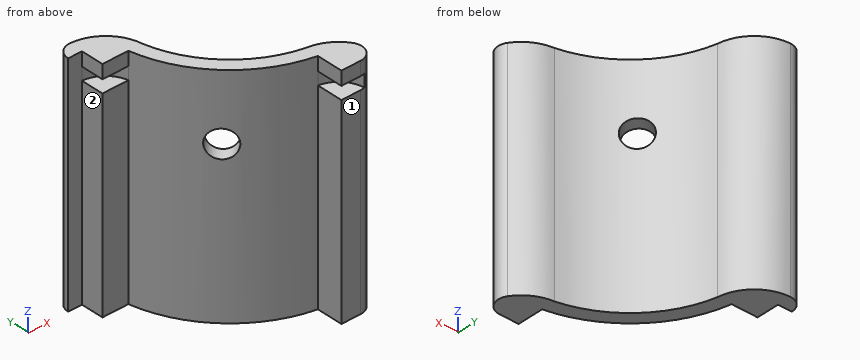
from build123d import *

# Parameters (mm, degrees)
BOSS_EXTRUDE1_DEPTH = 104.775
BOSS_EXTRUDE2_DEPTH = 92.5957
BOSS_EXTRUDE3_START = -5.8293
BOSS_EXTRUDE3_DEPTH = 5.8293
BOSS_EXTRUDE4_DEPTH = 6.35
SKETCH5_W           = 7.787485422
SKETCH5_H           = 19.833751934
SKETCH5_W_2         = 22.754058967
SKETCH5_H_2         = 3.407024872
CUT_EXTRUDE1_DEPTH  = 227.312030137
SKETCH6_R           = 6.35
CUT_EXTRUDE2_DEPTH  = 6.35
SKETCH7_W           = 111.054240747
SKETCH7_H           = 89.646194338
CUT_EXTRUDE3_DEPTH  = 104.775
SKETCH8_W           = 104.775
SKETCH8_H           = 6.354337814
BOSS_EXTRUDE5_DEPTH = 6.35
FILLET1_R           = 6.35


with BuildPart() as part:
    # Sketch1 → Boss-Extrude1 (new, symmetric)
    with BuildSketch(Plane.XY):
        with BuildLine():
            Line((-58.2422, 56.2102), (-58.2422, 62.5602))
            ThreePointArc((-58.2422, 62.5602), (-45.640852469, 57.743322347), (-39.3748699, 45.7962))
            ThreePointArc((-39.3748699, 45.7962), (-25.556268964, 20.239931036), (0, 6.4213301))
            ThreePointArc((0, 6.4213301), (12.247457496, 0.293755183), (17.272, -12.446))
            Line((17.272, -12.446), (10.922, -12.446))
            ThreePointArc((10.922, -12.446), (7.760938146, -4.204686933), (0, 0))
            ThreePointArc((0, 0), (-30.011530905, 15.784669095), (-45.7962, 45.7962))
            ThreePointArc((-45.7962, 45.7962), (-50.144819563, 53.243313205), (-58.2422, 56.2102))
        make_face()
    extrude(amount=BOSS_EXTRUDE1_DEPTH, both=True)


with BuildPart() as boss_extrude2_tool:
    # Sketch2 → Boss-Extrude2 (new, symmetric)
    with BuildSketch(Plane.XY):
        with BuildLine():
            Line((-58.2422, 56.2102), (-58.2422, 45.796198296))
            Line((-58.2422, 45.796198296), (-45.796199685, 45.796198296))
            ThreePointArc((-45.796199685, 45.796198296), (-50.144818899, 53.243312648), (-58.2422, 56.2102))
        make_face()
        with BuildLine():
            Line((0, 0), (0, -12.446))
            Line((0, -12.446), (10.922, -12.446))
            ThreePointArc((10.922, -12.446), (7.760938146, -4.204686933), (0, 0))
        make_face()
    extrude(amount=BOSS_EXTRUDE2_DEPTH, both=True)


with BuildPart() as part_1:
    add(part.part)


with BuildPart() as part_2:
    # Boss-Extrude2: joined with boss_extrude2_tool
    add(part_1.part.fuse(boss_extrude2_tool.part, tol=0.00001))

    # Sketch3 → Boss-Extrude3 (add)
    with BuildSketch(Plane(origin=(0, 0, -104.775), x_dir=(-1, 0, 0), z_dir=(0, 0, -1)).offset(BOSS_EXTRUDE3_START)):
        with BuildLine():
            Line((58.2422, 56.2102), (58.2422, 45.796198296))
            Line((58.2422, 45.796198296), (45.7962, 45.7962))
            ThreePointArc((45.7962, 45.7962), (50.144819563, 53.243313205), (58.2422, 56.2102))
        make_face()
        with BuildLine():
            Line((0, 0), (0, -12.446))
            Line((0, -12.446), (-10.922, -12.446))
            ThreePointArc((-10.922, -12.446), (-7.760938146, -4.204686933), (0, 0))
        make_face()
    extrude(amount=BOSS_EXTRUDE3_DEPTH)

    # Sketch4 → Boss-Extrude4 (add)
    with BuildSketch(Plane.XY.offset(104.775)):
        with BuildLine():
            Line((-58.2422, 56.2102), (-58.2422, 45.796198296))
            Line((-58.2422, 45.796198296), (-45.7962, 45.7962))
            ThreePointArc((-45.7962, 45.7962), (-50.144819563, 53.243313205), (-58.2422, 56.2102))
        make_face()
        with BuildLine():
            Line((0, 0), (0, -12.446))
            Line((0, -12.446), (10.922, -12.446))
            ThreePointArc((10.922, -12.446), (7.760938146, -4.204686933), (0, 0))
        make_face()
    extrude(amount=-BOSS_EXTRUDE4_DEPTH)

    # Sketch5 → Cut-Extrude1 (cut, through all)
    with BuildSketch(Plane.XY.offset(104.775)):
        with Locations((-61.627942711, 54.680509116)):
            Rectangle(SKETCH5_W, SKETCH5_H)
        with Locations((8.225058429, -13.641512436)):
            Rectangle(SKETCH5_W_2, SKETCH5_H_2)
    extrude(amount=-CUT_EXTRUDE1_DEPTH, mode=Mode.SUBTRACT)

    # Sketch6 → Cut-Extrude2 (cut, symmetric)
    with BuildSketch(Plane(origin=(-5.969, -5.969000176, 0), x_dir=(-0.7071067916239179, 0.7071067707491772, 0), z_dir=(-0.7071067707491772, -0.7071067916239179, 0))):
        with Locations(Location((32.382802858, -74.165398348, 0), (0, 0, 180))):
            Circle(SKETCH6_R)
    extrude(amount=CUT_EXTRUDE2_DEPTH, both=True, mode=Mode.SUBTRACT)

    # Sketch7 → Cut-Extrude3 (cut)
    with BuildSketch(Plane(origin=(0, 0, -104.775), x_dir=(-1, 0, 0), z_dir=(0, 0, -1))):
        with Locations((26.053941981, 26.416451063)):
            Rectangle(SKETCH7_W, SKETCH7_H)
    extrude(amount=-CUT_EXTRUDE3_DEPTH, mode=Mode.SUBTRACT)

    # Sketch8 → Boss-Extrude5 (add)
    with BuildSketch(Plane.ZY.offset(57.7342)):
        with Locations((52.3875, 59.374341949)):
            Rectangle(SKETCH8_W, SKETCH8_H)
    extrude(amount=BOSS_EXTRUDE5_DEPTH)

    # Fillet1
    # the kernel refuses this fillet: 6.35 mm, written as the material it takes off along each edge
    with BuildSketch(Plane(origin=(-64.0842, 62.551510856, -15.875), x_dir=(1, 0, 0), z_dir=(0, 0, 1))) as fillet1_piece_1:
        with BuildLine():
            CenterArc((FILLET1_R, -FILLET1_R), FILLET1_R, 90, 90)
            Line((0, -FILLET1_R), (0, 0))
            Line((0, 0), (FILLET1_R, 0))
        make_face()
    extrude(amount=136.525, mode=Mode.SUBTRACT)
    with BuildSketch(Plane(origin=(17.260151367, -11.938, -25.849178653), x_dir=(-0.30497213299383213, 0.9523612749882223, 0), z_dir=(0, 0, 1))) as fillet1_piece_2:
        with BuildLine():
            CenterArc((8.625598356, 6.114282737), FILLET1_R, 162.243512631, 123.416753829)
            Line((2.57810426, 8.050855782), (0, 0))
            ThreePointArc((0, 0), (5.169835731, -0.710949564), (10.339671461, 0))
        make_face()
    extrude(amount=156.473357306, mode=Mode.SUBTRACT)


solid = part_2.part
Work out the finished part from the listing and answer in its coordinate system (mm). Face numbers are marked on the shaded views. A direction names the side the tool comes from. Round coordinates to 2 decimals unless told otherwise and drop trailing zeros. Loops run counter-clockwise (first coordinate to the right, second up) from the corner with the lowest first, then second, coordinate; pieces in that order, holes last. Notation, with made-up numbers: (-16.75, 70.5) - (16.25, 70.5) arc R8 cw to (16.25, 83.5) - close; hole circle Ø9 at (53.5, 63). An arc over 180 degrees is marked (long way). One line per item, written item: value.
Q1. For the marked faces 1 and 2, determine the directions among +Z, -Z, +X, -X, +Y, -Y from which every point of the face is accessible in a straight line to the end or side of a thin tool.
Check values:
face 1: +Z, -Z, +X, -X, -Y
face 2: +Z, -Z, -X, -Y
Q2. Straight lines are drawn through the part: probe 1 along Y at (x, z) = (-23.5, 54); probe 2 along Y at (x, z) = (-35, 32.5); probe 3 along X at (y, z) = (37.5, 88). For each, find the intervals that lie inside material, in ascending order.
Check values:
probe 1: 10.19 to 18.3
probe 2: 21.48 to 33.29
probe 3: -43.61 to -36.89
Q3. Find section B-B on x = -48. Give the vertices of the cut face in (y, z) (3 decimals).
Check values:
outline: (45.796, 0) - (59.532, 0) - (59.532, 104.775) - (45.796, 104.775) - (45.796, 98.425) - (50.942, 98.425) - (50.942, 92.596) - (45.796, 92.596) - close
Q4. Find section C-C on y = 52.5. Give the vertices of the cut face in (x, z) (3 decimals), and give its area (3 significant figures).
Check values:
outline: (-57.734, 0) - (-41.501, 0) - (-41.501, 104.775) - (-57.734, 104.775) - (-57.734, 98.425) - (-49.331, 98.425) - (-49.331, 92.596) - (-57.734, 92.596) - close
area: 1,650 mm2
Q5. Each of these flat-tipped pins is pushed along its axis until it touches: pin 1 Ø5 at (y, z) = (49, 100.5) entering from -X; pin 2 Ø3.5 at (x, z) = (-51, 57) entering from -Y; pin 3 Ø12 at (x, y) = (4.5, -7.5) entering from -Z; pin 4 Ø10 at (y, z) = (41, 40.5) entering from +X. Where does it stop, or does it pass through?
Check values:
pin 1: x = -57.73
pin 2: y = 45.8
pin 3: z = 0
pin 4: x = -36.27
Q6. Find section D-D on y = 31. Give the vertices of the cut face in (x, z) (1 decimal).
Check values:
outline: (-40.9, 0) - (-33.8, 0) - (-33.8, 104.8) - (-40.9, 104.8) - close
